Input: part model. Units: mm. Frame: model coordinates. Face numbers are marked on the shaded views. A direction names the side the tool comes from. Coordinates: 2 decimals unless noted, no trailing zeros. Write each loop counter-clockwise with the first axis right and the second up, starting at its lowest first coordinate (ties: lowest second). Pieces come first, ordered by that corner, then holes. Notation, with made-up numbers: (79, 6.5) - (108, 6.5) arc R30 ccw to (108, 41.5) - close; hole circle Ø6 at (87.5, 46). An arc over 180 degrees is marked (long way). Put each result on its own line as item: value. Start each with the question number.
1. Cut plane A-A, the plane z = 25. Return loops of the section in (x, y), and give its area (3 significant figures).
2. Cut plane D-D, the plane y = 12. Return loops of the section in (x, z).
3. Cut plane C-C, the plane x = 1.5. Return loops of the section in (y, z), and give its area (3 significant figures).
4. Pin query (flat end, axial travel): pin 1 (11.5 mm diameter, centred on x = 0.5, y = 5.5, fed in from +Z); pin 2 (1.5 mm diameter, centred on x = -19, z = 33.5, fed in from -Y); pin 3 (3 mm diameter, centred on x = 14.5, z = 8, fed in from -Y). Return the tip coordinate at first contact, or that it passes through.
5. Access query for the marked faces 1 and 2. Directions: +Z, -Z, +X, -X, +Y, -Y. A direction counts if a zero-diameter tool reaches every point of the face in a straight line with its end or side. Return the directions, or none.
6. Cut plane B-B, the plane y = 0. Return loops of the section in (x, z).
7. Line query: line 1 (Y direction, x = 0, z = 4); line 2 (X direction, y = -2.5, z = 8.5); line 3 (Z direction, x = -5, y = 13). Output: solid intervals per line, ascending.
8. Pull-direction query (X, two-part tool) for the marked faces 3, 4 and 5; classes: released by +X, released by -X, zero draft, split by the parting line, or undercut.
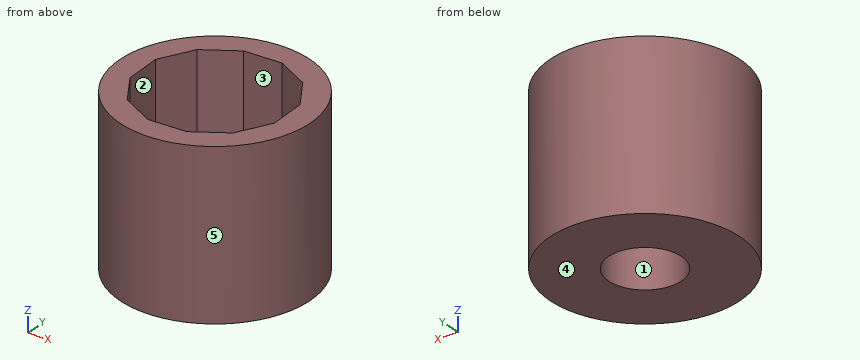
from build123d import *

# Parameters (mm, degrees)
F0_R     = 26
F0_R_2   = 10
F1_DEPTH = 20
F2_R     = 26
F3_DEPTH = 25


with BuildPart() as f1:
    # F0 (on Top) → F1 (new body)
    with BuildSketch(Plane.XY):
        Circle(F0_R)
        Circle(F0_R_2, mode=Mode.SUBTRACT)
    extrude(amount=F1_DEPTH)

    # F2 (on face) → F3 (join)
    with BuildSketch(Plane.XY.offset(20)):
        Circle(F2_R)
        with BuildLine():
            ThreePointArc((19.016501, 6.194569), (19.752595, 3.136078), (20, 0))
            ThreePointArc((20, 0), (19.891219, -2.083129), (19.566057, -4.143597))
            ThreePointArc((19.566057, -4.143597), (17.826918, -9.066476), (14.872904, -13.371489))
            ThreePointArc((14.872904, -13.371489), (10.905326, -16.765257), (6.194569, -19.016501))
            ThreePointArc((6.194569, -19.016501), (1.061661, -19.971802), (-4.143597, -19.566057))
            ThreePointArc((-4.143597, -19.566057), (-9.066476, -17.826918), (-13.371489, -14.872904))
            ThreePointArc((-13.371489, -14.872904), (-16.765257, -10.905326), (-19.016501, -6.194569))
            ThreePointArc((-19.016501, -6.194569), (-19.971802, -1.061661), (-19.566057, 4.143597))
            ThreePointArc((-19.566057, 4.143597), (-17.826918, 9.066476), (-14.872904, 13.371489))
            ThreePointArc((-14.872904, 13.371489), (-10.905326, 16.765257), (-6.194569, 19.016501))
            ThreePointArc((-6.194569, 19.016501), (-1.061661, 19.971802), (4.143597, 19.566057))
            ThreePointArc((4.143597, 19.566057), (9.066476, 17.826918), (13.371489, 14.872904))
            ThreePointArc((13.371489, 14.872904), (16.765257, 10.905326), (19.016501, 6.194569))
        make_face(mode=Mode.SUBTRACT)
        with BuildLine():
            Line((-14.872904, 13.371489), (-6.194569, 19.016501))
            ThreePointArc((-6.194569, 19.016501), (-10.905326, 16.765257), (-14.872904, 13.371489))
        make_face()
        with BuildLine():
            Line((-6.194569, 19.016501), (4.143597, 19.566057))
            ThreePointArc((4.143597, 19.566057), (-1.061661, 19.971802), (-6.194569, 19.016501))
        make_face()
        with BuildLine():
            Line((4.143597, 19.566057), (13.371489, 14.872904))
            ThreePointArc((13.371489, 14.872904), (9.066476, 17.826918), (4.143597, 19.566057))
        make_face()
        with BuildLine():
            Line((13.371489, 14.872904), (19.016501, 6.194569))
            ThreePointArc((19.016501, 6.194569), (16.765257, 10.905326), (13.371489, 14.872904))
        make_face()
        with BuildLine():
            Line((-19.566057, 4.143597), (-14.872904, 13.371489))
            ThreePointArc((-14.872904, 13.371489), (-17.826918, 9.066476), (-19.566057, 4.143597))
        make_face()
        with BuildLine():
            ThreePointArc((-13.371489, -14.872904), (-9.066476, -17.826918), (-4.143597, -19.566057))
            Line((-4.143597, -19.566057), (-13.371489, -14.872904))
        make_face()
        with BuildLine():
            ThreePointArc((-19.016501, -6.194569), (-16.765257, -10.905326), (-13.371489, -14.872904))
            Line((-13.371489, -14.872904), (-19.016501, -6.194569))
        make_face()
        with BuildLine():
            ThreePointArc((-4.143597, -19.566057), (1.061661, -19.971802), (6.194569, -19.016501))
            Line((6.194569, -19.016501), (-4.143597, -19.566057))
        make_face()
        with BuildLine():
            ThreePointArc((6.194569, -19.016501), (10.905326, -16.765257), (14.872904, -13.371489))
            Line((14.872904, -13.371489), (6.194569, -19.016501))
        make_face()
        with BuildLine():
            ThreePointArc((14.872904, -13.371489), (17.826918, -9.066476), (19.566057, -4.143597))
            Line((19.566057, -4.143597), (14.872904, -13.371489))
        make_face()
        with BuildLine():
            ThreePointArc((19.566057, -4.143597), (19.891219, -2.083129), (20, 0))
            ThreePointArc((20, 0), (19.752595, 3.136078), (19.016501, 6.194569))
            Line((19.016501, 6.194569), (19.566057, -4.143597))
        make_face()
        with BuildLine():
            Line((-19.016501, -6.194569), (-19.566057, 4.143597))
            ThreePointArc((-19.566057, 4.143597), (-19.971802, -1.061661), (-19.016501, -6.194569))
        make_face()
    extrude(amount=F3_DEPTH)


solid = f1.part
Report:
1. outline: circle Ø52 at (0, 0); hole (-19.57, 4.14) - (-19.02, -6.19) - (-13.37, -14.87) - (-4.14, -19.57) - (6.19, -19.02) - (14.87, -13.37) - (19.57, -4.14) - (19.02, 6.19) - (13.37, 14.87) - (4.14, 19.57) - (-6.19, 19.02) - (-14.87, 13.37) - close
1. area: 924 mm^2
2. outline: (-23.07, 0) - (23.07, 0) - (23.07, 45) - (15.24, 45) - (15.24, 20) - (-15.57, 20) - (-15.57, 45) - (-23.07, 45) - close
3. outline: (-25.96, 0) - (-9.89, 0) - (-9.89, 20) - (-19.27, 20) - (-19.27, 45) - (-25.96, 45) - close; (9.89, 0) - (25.96, 0) - (25.96, 45) - (19.43, 45) - (19.43, 20) - (9.89, 20) - close
3. area: 973 mm^2
4. pin 1: stops at z = 20
4. pin 2: stops at y = -18.52
4. pin 3: stops at y = -22.52
5. face 1: +Z, -Z
5. face 2: +Z
6. outline: (-26, 0) - (-10, 0) - (-10, 20) - (-19.35, 20) - (-19.35, 45) - (-26, 45) - close; (10, 0) - (26, 0) - (26, 45) - (19.35, 45) - (19.35, 20) - (10, 20) - close
7. line 1: y = -26 to -10, 10 to 26
7. line 2: x = -25.88 to -9.68, 9.68 to 25.88
7. line 3: z = 0 to 20
8. face 3: undercut
8. face 4: zero draft
8. face 5: split by the parting line
